```python
from build123d import *

# Parameters (mm, degrees)
SKETCH1_R           = 2.125
BOSS_EXTRUDE1_DEPTH = 2
BOSS_EXTRUDE2_DEPTH = 0.5


with BuildPart() as part:
    # Sketch1 → Boss-Extrude1 (new body)
    with BuildSketch(Plane.XY):
        with BuildLine():
            Line((-64.378174593, 10.621320344), (-62.656854249, 8.9))
            Line((-62.656854249, 8.9), (-62.656854249, 8.585786438))
            ThreePointArc((-62.656854249, 8.585786438), (-62.428492847, 7.437736141), (-61.778174593, 6.464466094))
            Line((-61.778174593, 6.464466094), (-56.192388155, 0.878679656))
            ThreePointArc((-56.192388155, 0.878679656), (-55.219118109, 0.228361402), (-54.071067812, 0))
            Line((-54.071067812, 0), (-1.242640687, 0))
            ThreePointArc((-1.242640687, 0), (-0.09459039, 0.228361402), (0.878679656, 0.878679656))
            Line((0.878679656, 0.878679656), (6.464466094, 6.464466094))
            ThreePointArc((6.464466094, 6.464466094), (7.114784348, 7.437736141), (7.343145751, 8.585786438))
            Line((7.343145751, 8.585786438), (7.343145751, 8.9))
            Line((7.343145751, 8.9), (9.064466094, 10.621320344))
            ThreePointArc((9.064466094, 10.621320344), (9.714784348, 11.59459039), (9.943145751, 12.742640687))
            Line((9.943145751, 12.742640687), (9.943145751, 40.257359313))
            ThreePointArc((9.943145751, 40.257359313), (9.714784348, 41.40540961), (9.064466094, 42.378679656))
            Line((9.064466094, 42.378679656), (7.343145751, 44.1))
            Line((7.343145751, 44.1), (7.343145751, 44.414213562))
            ThreePointArc((7.343145751, 44.414213562), (7.114784348, 45.562263859), (6.464466094, 46.535533906))
            Line((6.464466094, 46.535533906), (0.878679656, 52.121320344))
            ThreePointArc((0.878679656, 52.121320344), (-0.09459039, 52.771638598), (-1.242640687, 53))
            Line((-1.242640687, 53), (-54.071067812, 53))
            ThreePointArc((-54.071067812, 53), (-55.219118109, 52.771638598), (-56.192388155, 52.121320344))
            Line((-56.192388155, 52.121320344), (-61.778174593, 46.535533906))
            ThreePointArc((-61.778174593, 46.535533906), (-62.428492847, 45.562263859), (-62.656854249, 44.414213562))
            Line((-62.656854249, 44.414213562), (-62.656854249, 44.1))
            Line((-62.656854249, 44.1), (-64.378174593, 42.378679656))
            ThreePointArc((-64.378174593, 42.378679656), (-65.028492847, 41.40540961), (-65.256854249, 40.257359313))
            Line((-65.256854249, 40.257359313), (-65.256854249, 12.742640687))
            ThreePointArc((-65.256854249, 12.742640687), (-65.028492847, 11.59459039), (-64.378174593, 10.621320344))
        make_face()
        with Locations((4.443145751, 37.5)):
            Circle(SKETCH1_R, mode=Mode.SUBTRACT)
        with Locations((-59.756854249, 37.5)):
            Circle(SKETCH1_R, mode=Mode.SUBTRACT)
        with Locations((-59.756854249, 15.5)):
            Circle(SKETCH1_R, mode=Mode.SUBTRACT)
        with Locations((4.443145751, 15.5)):
            Circle(SKETCH1_R, mode=Mode.SUBTRACT)
        with BuildLine():
            Line((-1.656854249, 49), (-53.656854249, 49))
            Line((-53.656854249, 49), (-58.656854249, 44))
            Line((-58.656854249, 44), (-58.656854249, 43.398304841))
            ThreePointArc((-58.656854249, 43.398304841), (-55.141661946, 41.334057903), (-53.756854249, 37.5))
            Line((-53.756854249, 37.5), (-53.756854249, 15.5))
            ThreePointArc((-53.756854249, 15.5), (-55.141661946, 11.665942097), (-58.656854249, 9.601695159))
            Line((-58.656854249, 9.601695159), (-58.656854249, 9))
            Line((-58.656854249, 9), (-53.656854249, 4))
            Line((-53.656854249, 4), (-1.656854249, 4))
            Line((-1.656854249, 4), (3.343145751, 9))
            Line((3.343145751, 9), (3.343145751, 9.601695159))
            ThreePointArc((3.343145751, 9.601695159), (-0.172046553, 11.665942097), (-1.556854249, 15.5))
            Line((-1.556854249, 15.5), (-1.556854249, 37.5))
            ThreePointArc((-1.556854249, 37.5), (-0.172046553, 41.334057903), (3.343145751, 43.398304841))
            Line((3.343145751, 43.398304841), (3.343145751, 44))
            Line((3.343145751, 44), (-1.656854249, 49))
        make_face(mode=Mode.SUBTRACT)
    extrude(amount=BOSS_EXTRUDE1_DEPTH)

    # Sketch2 → Boss-Extrude2 (add)
    with BuildSketch(Plane.XY.offset(2)):
        with BuildLine():
            Line((-62.156854249, 9.107106781), (-62.156854249, 8.585786438))
            ThreePointArc((-62.156854249, 8.585786438), (-61.966553081, 7.629077857), (-61.424621202, 6.818019485))
            Line((-61.424621202, 6.818019485), (-55.838834765, 1.232233047))
            ThreePointArc((-55.838834765, 1.232233047), (-55.027776393, 0.690301169), (-54.071067812, 0.5))
            Line((-54.071067812, 0.5), (-1.242640687, 0.5))
            ThreePointArc((-1.242640687, 0.5), (-0.285932106, 0.690301169), (0.525126266, 1.232233047))
            Line((0.525126266, 1.232233047), (6.110912703, 6.818019485))
            ThreePointArc((6.110912703, 6.818019485), (6.652844582, 7.629077857), (6.843145751, 8.585786438))
            Line((6.843145751, 8.585786438), (6.843145751, 9.107106781))
            Line((6.843145751, 9.107106781), (8.710912703, 10.974873734))
            ThreePointArc((8.710912703, 10.974873734), (9.252844582, 11.785932106), (9.443145751, 12.742640687))
            Line((9.443145751, 12.742640687), (9.443145751, 40.257359313))
            ThreePointArc((9.443145751, 40.257359313), (9.252844582, 41.214067894), (8.710912703, 42.025126266))
            Line((8.710912703, 42.025126266), (6.843145751, 43.892893219))
            Line((6.843145751, 43.892893219), (6.843145751, 44.414213562))
            ThreePointArc((6.843145751, 44.414213562), (6.652844582, 45.370922143), (6.110912703, 46.181980515))
            Line((6.110912703, 46.181980515), (0.525126266, 51.767766953))
            ThreePointArc((0.525126266, 51.767766953), (-0.285932106, 52.309698831), (-1.242640687, 52.5))
            Line((-1.242640687, 52.5), (-54.071067812, 52.5))
            ThreePointArc((-54.071067812, 52.5), (-55.027776393, 52.309698831), (-55.838834765, 51.767766953))
            Line((-55.838834765, 51.767766953), (-61.424621202, 46.181980515))
            ThreePointArc((-61.424621202, 46.181980515), (-61.966553081, 45.370922143), (-62.156854249, 44.414213562))
            Line((-62.156854249, 44.414213562), (-62.156854249, 43.892893219))
            Line((-62.156854249, 43.892893219), (-64.024621202, 42.025126266))
            ThreePointArc((-64.024621202, 42.025126266), (-64.566553081, 41.214067894), (-64.756854249, 40.257359313))
            Line((-64.756854249, 40.257359313), (-64.756854249, 12.742640687))
            ThreePointArc((-64.756854249, 12.742640687), (-64.566553081, 11.785932106), (-64.024621202, 10.974873734))
            Line((-64.024621202, 10.974873734), (-62.156854249, 9.107106781))
        make_face()
        with BuildLine():
            Line((-61.156854249, 9.521320344), (-61.156854249, 8.585786438))
            ThreePointArc((-61.156854249, 8.585786438), (-61.042673548, 8.011761289), (-60.717514421, 7.525126266))
            Line((-60.717514421, 7.525126266), (-55.131727984, 1.939339828))
            ThreePointArc((-55.131727984, 1.939339828), (-54.64509296, 1.614180701), (-54.071067812, 1.5))
            Line((-54.071067812, 1.5), (-1.242640687, 1.5))
            ThreePointArc((-1.242640687, 1.5), (-0.668615539, 1.614180701), (-0.181980515, 1.939339828))
            Line((-0.181980515, 1.939339828), (5.403805922, 7.525126266))
            ThreePointArc((5.403805922, 7.525126266), (5.728965049, 8.011761289), (5.843145751, 8.585786438))
            Line((5.843145751, 8.585786438), (5.843145751, 9.521320344))
            Line((5.843145751, 9.521320344), (8.003805922, 11.681980515))
            ThreePointArc((8.003805922, 11.681980515), (8.328965049, 12.168615539), (8.443145751, 12.742640687))
            Line((8.443145751, 12.742640687), (8.443145751, 40.257359313))
            ThreePointArc((8.443145751, 40.257359313), (8.328965049, 40.831384461), (8.003805922, 41.318019485))
            Line((8.003805922, 41.318019485), (5.843145751, 43.478679656))
            Line((5.843145751, 43.478679656), (5.843145751, 44.414213562))
            ThreePointArc((5.843145751, 44.414213562), (5.728965049, 44.988238711), (5.403805922, 45.474873734))
            Line((5.403805922, 45.474873734), (-0.181980515, 51.060660172))
            ThreePointArc((-0.181980515, 51.060660172), (-0.668615539, 51.385819299), (-1.242640687, 51.5))
            Line((-1.242640687, 51.5), (-54.071067812, 51.5))
            ThreePointArc((-54.071067812, 51.5), (-54.64509296, 51.385819299), (-55.131727984, 51.060660172))
            Line((-55.131727984, 51.060660172), (-60.717514421, 45.474873734))
            ThreePointArc((-60.717514421, 45.474873734), (-61.042673548, 44.988238711), (-61.156854249, 44.414213562))
            Line((-61.156854249, 44.414213562), (-61.156854249, 43.478679656))
            Line((-61.156854249, 43.478679656), (-63.317514421, 41.318019485))
            ThreePointArc((-63.317514421, 41.318019485), (-63.642673548, 40.831384461), (-63.756854249, 40.257359313))
            Line((-63.756854249, 40.257359313), (-63.756854249, 12.742640687))
            ThreePointArc((-63.756854249, 12.742640687), (-63.642673548, 12.168615539), (-63.317514421, 11.681980515))
            Line((-63.317514421, 11.681980515), (-61.156854249, 9.521320344))
        make_face(mode=Mode.SUBTRACT)
    extrude(amount=BOSS_EXTRUDE2_DEPTH)


solid = part.part
```
Could you check a few things on this model? Use its own coordinates, in mm. A direction names the side the tool comes from. Coordinates: 2 decimals unless noted, no trailing zeros. Write each loop counter-clockwise with the first axis right and the second up, starting at its lowest first coordinate (ties: lowest second). Pieces come first, ordered by that corner, then holes. Notation, with made-up numbers: (8.5, 40.5) -> (53.5, 40.5) arc R24 cw to (53.5, 61.5) -> close; hole circle Ø3 at (-23, 30). An arc over 180 degrees is marked (long way). Return JSON: item names as keys, results as strings.
(1) We'd pull the mould along Y, two halves only. Please class faces 6 (the flat face through (-27, 49, 1)), 7 (the flat face through (-25, 3, 0)), 8 (the cylindrical face through (-62.42, 45.58, 0.99)): +Y half, -Y half, draft (parallel to the pull), parting line (faces both ways), or undercut.
Numbers:
{"face 6": "undercut", "face 7": "draft", "face 8": "+Y half"}
(2) I need wall thicknesses on L1, parallel to Y at x = -30, z = 1.4; L2, parallel to Y at x = 0.5, z = 0.35; L3, parallel to Y at x = -59, z = 1.7. Which ranges of each line are inside material? Lowest first, please.
Numbers:
{"L1": "y = 0 to 4, 49 to 53", "L2": "y = 0.56 to 6.16, 10.98 to 42.02, 46.84 to 52.44", "L3": "y = 3.69 to 13.51, 17.49 to 35.51, 39.49 to 49.31"}
(3) I'm going to push a flat-ended pin straight in: pin 1 (5.5 mm diameter, centred on x = -59.76, y = 15.5, fed in from +Z). Where does the tip first touch, or does it pass through?
Numbers:
{"pin 1": "stops at z = 2"}
(4) Which directions (+Z, -Z, +X, -X, +Y, -Y) give clear straight access to the entire face, cutting with the end or side of a thin tool? Please do faces 1 (the cylindrical face through (-0.079, 52.765, 0.986)), 2 (the flat face through (3.279, 3.986, 2.246)), 3 (the flat face through (-28, 51, 2)), 4 (the cylindrical face through (-0.11, 0.22, 0.99)), 5 (the flat face through (-56.122, 46.535, 0.986)).
Numbers:
{"face 1": "+Z, -Z, +X, +Y", "face 2": "+Z, +X, -Y", "face 3": "+Z", "face 4": "+Z, -Z, +X, -Y", "face 5": "+Z, -Z"}
(5) Imagine slicing it at C-C, the plane z = 0.5. Count the separate pieces of the cut face and the enclosed holes in it, then the cut area to 3 significant figures.
Numbers:
{"separate pieces": "1", "enclosed holes": "5", "area": "1,280 mm2"}
(6) Imagine slicing it at A-A, the plane x = -50.5. Please give me the cut outline in (y, z), then the cut area to 3 significant figures.
Numbers:
{"outline": "(0, 0) -> (4, 0) -> (4, 2) -> (1.5, 2) -> (1.5, 2.5) -> (0.5, 2.5) -> (0.5, 2) -> (0, 2) -> close; (49, 0) -> (53, 0) -> (53, 2) -> (52.5, 2) -> (52.5, 2.5) -> (51.5, 2.5) -> (51.5, 2) -> (49, 2) -> close", "area": "17.0 mm2"}
(7) Imagine slicing it at B-B, the plane y = 33. Please give me the cut outline in (x, z), then the cut area to 3 significant figures.
Numbers:
{"outline": "(-65.26, 0) -> (-53.76, 0) -> (-53.76, 2) -> (-63.76, 2) -> (-63.76, 2.5) -> (-64.76, 2.5) -> (-64.76, 2) -> (-65.26, 2) -> close; (-1.56, 0) -> (9.94, 0) -> (9.94, 2) -> (9.44, 2) -> (9.44, 2.5) -> (8.44, 2.5) -> (8.44, 2) -> (-1.56, 2) -> close", "area": "47.0 mm2"}
